Can you work these out from the model? Positions are in its coordinate system, mm. A direction names the side the tool comes from. Round coordinates to 2 decimals unless told otherwise and drop trailing zeros. Loops run counter-clockwise (first coordinate to the right, second up) from the corner with the lowest first, then second, coordinate; pieces in that order, holes last. Notation, with made-up numbers: (89.25, 45.25) -> (128.25, 45.25) arc R17 cw to (128.25, 58.25) -> close; hole circle Ø10 at (19, 76.5). An arc over 180 degrees is marked (long way). Write each question's results on one line, items separated by ' | '.
from build123d import *

# Parameters (mm, degrees)
SKETCH1_W           = 509
SKETCH1_H           = 605
BOSS_EXTRUDE1_DEPTH = 0.8
SKETCH2_W           = 20
SKETCH2_H           = 100
BOSS_EXTRUDE2_DEPTH = 0.8
SKETCH4_W           = 20
SKETCH4_H           = 100
BOSS_EXTRUDE3_DEPTH = 0.8
SKETCH5_W           = 20
SKETCH5_H           = 100
BOSS_EXTRUDE4_DEPTH = 0.8


with BuildPart() as part:
    # Sketch1 → Boss-Extrude1 (new body)
    with BuildSketch(Plane.XY):
        with Locations((254.5, 302.5)):
            Rectangle(SKETCH1_W, SKETCH1_H)
    extrude(amount=BOSS_EXTRUDE1_DEPTH)

    # Sketch2 → Boss-Extrude2 (add)
    with BuildSketch(Plane.XY.offset(0.8)):
        with Locations((10, 342.918789735)):
            Rectangle(SKETCH2_W, SKETCH2_H)
        with Locations((499, 342.918789735)):
            Rectangle(SKETCH2_W, SKETCH2_H)
    extrude(amount=BOSS_EXTRUDE2_DEPTH)

    # Sketch4 → Boss-Extrude3 (add)
    with BuildSketch(Plane.ZY):
        with Locations((11.6, 342.918789735)):
            Rectangle(SKETCH4_W, SKETCH4_H)
    extrude(amount=-BOSS_EXTRUDE3_DEPTH)

    # Sketch5 → Boss-Extrude4 (add)
    with BuildSketch(Plane(origin=(509, 0, 0), x_dir=(0, 0, -1), z_dir=(1, 0, 0))):
        with Locations((-11.6, 342.918789735)):
            Rectangle(SKETCH5_W, SKETCH5_H)
    extrude(amount=-BOSS_EXTRUDE4_DEPTH)


solid = part.part
1. If we section it at B-B (y = 325): List the corners of the cut face in (x, z) for me.
Final values:
outline: (0, 0) -> (509, 0) -> (509, 21.6) -> (508.2, 21.6) -> (508.2, 1.6) -> (489, 1.6) -> (489, 0.8) -> (20, 0.8) -> (20, 1.6) -> (0.8, 1.6) -> (0.8, 21.6) -> (0, 21.6) -> close
2. If we section it at D-D (y = 107.5): List the corners of the cut face in (x, z) for me, then the cut area to 3 significant figures.
Final values:
outline: (0, 0) -> (509, 0) -> (509, 0.8) -> (0, 0.8) -> close | area: 407 mm2
3. If we section it at A-A (z = 6.75): List the corners of the cut face in (x, y) for me, then the cut area to 3 significant figures.
Final values:
outline: (0, 292.92) -> (0.8, 292.92) -> (0.8, 392.92) -> (0, 392.92) -> close; (508.2, 292.92) -> (509, 292.92) -> (509, 392.92) -> (508.2, 392.92) -> close | area: 160 mm2
4. We'd pull the mould along X, two halves only. Please class faces 1 (the face through (251, 307, 0)), 2 (the face through (0.8, 344, 11)), 3 (the face through (509, 326, 9)): pulls with the +X half, pulls with the -X half, needs draft (parallel to the pull), parting line crosses it, or undercut.
Final values:
face 1: needs draft | face 2: undercut | face 3: pulls with the +X half
5. If we section it at C-C (x = 224.5): List the corners of the cut face in (y, z) for me.
Final values:
outline: (0, 0) -> (605, 0) -> (605, 0.8) -> (0, 0.8) -> close
6. Please list where these lines run through material, in increasing order: line 1 (X direction, y = 293, z = 13); line 2 (Z direction, x = 466, y = 467); line 3 (X direction, y = 385, z = 1.5). Write a range as from..to.
Final values:
line 1: 0..0.8, 508.2..509 | line 2: 0..0.8 | line 3: 0..20, 489..509
7. Will these pins go through, and if not, where does the flat tip stop? pin 1 (21 mm diameter, centred on x = 8.5, y = 325, fed in from +Z); pin 2 (6 mm diameter, centred on x = 497, y = 360, fed in from +Z); pin 3 (10 mm diameter, centred on x = 74, y = 433, fed in from +Z); pin 4 (10 mm diameter, centred on x = 9.5, z = 12.5, fed in from -Y).
Final values:
pin 1: z = 21.6 | pin 2: z = 1.6 | pin 3: z = 0.8 | pin 4: through
8. On a 3-axis mill with a long thin cutter (end or side, diameter ignored), from which of +Z, -Z, +X, -X, +Y, -Y can I reach the whole of each face in a straight line? I mean faces 4 (the face through (508.7, 392.919, 6.6)), 5 (the face through (508.7, 292.919, 6.6)), 6 (the face through (10, 344, 1.6)). Say none if no direction works.
Final values:
face 4: +Z, +X, -X, +Y | face 5: +Z, +X, -X, -Y | face 6: +Z, +Y, -Y
